Answer from the drawing. Dimensions are ordinates in mm from the lowest x, y and z of the part. Round coordinates to 2 decimals unless told otherwise and drop trailing zeros. Order: outer loops, then holes, each group sorted by start corner. A loop starts at its lowest first (then second) coordinate and runs counter-clockwise, first axis right, second up. Notation, with made-up numbers: (7, 45) -> (47, 45) arc R25 ccw to (47, 64) -> close; hole circle Ø11 at (9, 35). An arc over 180 degrees is marked (long way). Use a Markdown table: item, result. Add a question column.
Item 1: A cutting plane is placed at A-A, the plane x = 18. Determine the outline of the cut face in (y, z).
Item 2: A cutting plane is placed at C-C, the plane z = 153. Determine the outline of the cut face in (x, y), plus the area to 3 significant figures.
Item 3: Find the intervals of material crossed by L1, parallel to X at y = 1.85, z = 100; L2, parallel to X at y = 3.1, z = 146, in increasing order. Write a range as [from, to].
Item 4: A cutting plane is placed at B-B, the plane y = 4.2. Determine the outline of the cut face in (x, z).
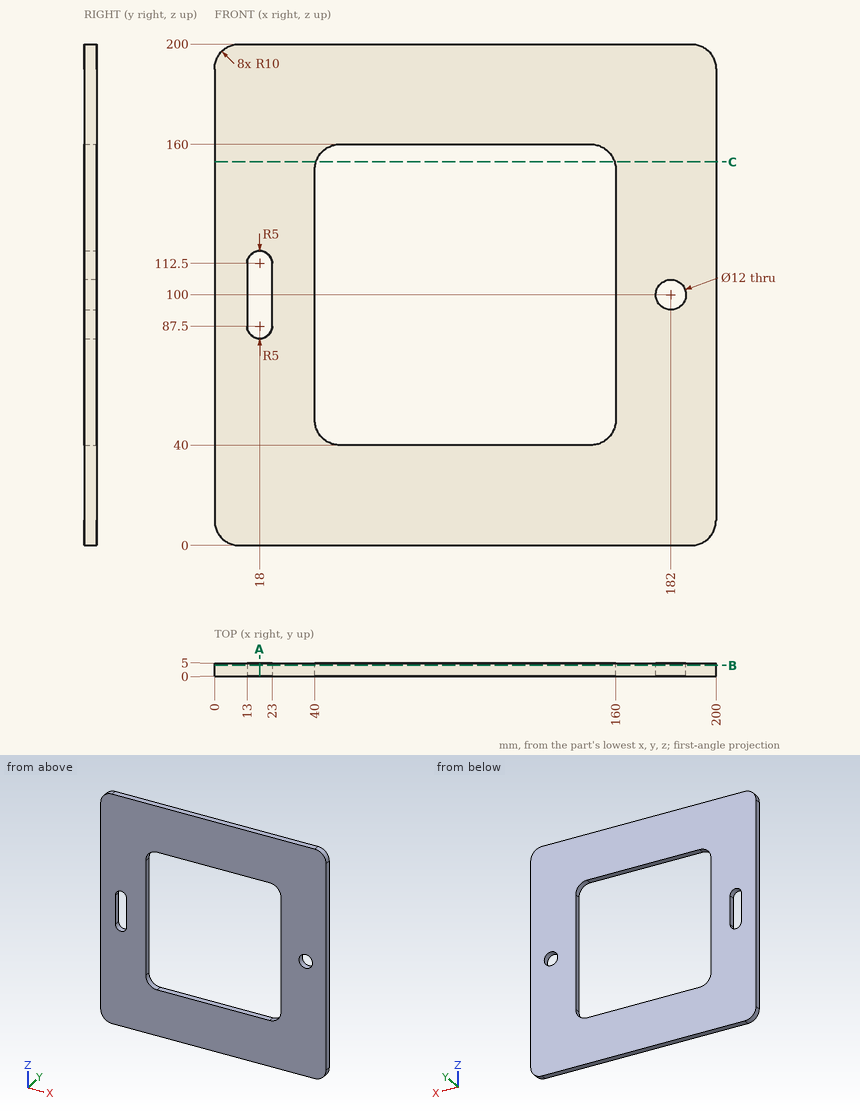
Reported:
| question | item | result |
|---|---|---|
| 1 | outline | (0, 0) -> (5, 0) -> (5, 82.5) -> (0, 82.5) -> close; (0, 117.5) -> (5, 117.5) -> (5, 200) -> (0, 200) -> close |
| 2 | outline | (0, 0) -> (40.46, 0) -> (40.46, 5) -> (0, 5) -> close; (159.54, 0) -> (200, 0) -> (200, 5) -> (159.54, 5) -> close |
| 2 | area | 405 mm² |
| 3 | L1 | [0, 13], [23, 40], [160, 176], [188, 200] |
| 3 | L2 | [0, 40], [160, 200] |
| 4 | outline | (0, 10) arc R10 ccw to (10, 0) -> (190, 0) arc R10 ccw to (200, 10) -> (200, 190) arc R10 ccw to (190, 200) -> (10, 200) arc R10 ccw to (0, 190) -> close; hole (13, 87.5) arc R5 ccw to (23, 87.5) -> (23, 112.5) arc R5 ccw to (13, 112.5) -> close; hole (40, 50) arc R10 ccw to (50, 40) -> (150, 40) arc R10 ccw to (160, 50) -> (160, 150) arc R10 ccw to (150, 160) -> (50, 160) arc R10 ccw to (40, 150) -> close; hole circle Ø12 at (182, 100) |
